Could you check a few things on this model? Use its own coordinates, in mm. A direction names the side the tool comes from. Coordinates: 2 decimals unless noted, no trailing zeros. Order: outer loops, then holes, each group sorted by start corner. A loop starts at its lowest first (then second) coordinate and runs counter-clockwise, first axis right, second up. Notation, with made-up numbers: M 28.5,22 L 86.5,22 A22 cw 86.5,33 Z; hole C -8,47.5 d8. An arc over 180 degrees is marked long. One line per question, with ' | ' between items. Start each with the question number.
from build123d import *

# Parameters (mm, degrees)
F0_R     = 28.575
F1_DEPTH = 40.2336
F2_R     = 3.302
F3_R     = 10.16
F4_DEPTH = 15.7734


with BuildPart() as f1:
    # F0 (on Top) → F1 (new body)
    with BuildSketch(Plane.XY):
        Circle(F0_R)
        with BuildLine():
            ThreePointArc((13.4477648793, -4.826), (-14.2875, 0), (13.4477648793, 4.826))
            Line((13.4477648793, 4.826), (18.5293, 4.826))
            Line((18.5293, 4.826), (18.5293, -4.826))
            Line((18.5293, -4.826), (13.4477648793, -4.826))
        make_face(mode=Mode.SUBTRACT)
    extrude(amount=F1_DEPTH)

    # F2
    f2_edges = [f1.edges().sort_by_distance(p)[0] for p in [
        (-28.575, 0, 40.2336),
    ]]
    fillet(f2_edges, radius=F2_R)

    # F3 (on face) → F4 (join)
    with BuildSketch(Plane(origin=(0, 0, 0), x_dir=(1, 0, 0), z_dir=(0, 0, -1))):
        with BuildLine():
            Line((5.7964106128, -27.9809265216), (57.1919272622, -18.7764181619))
            ThreePointArc((57.1919272622, -18.7764181619), (73.025, 0), (57.1919272622, 18.7764181619))
            Line((57.1919272622, 18.7764181619), (5.7964106128, 27.9809265216))
            ThreePointArc((5.7964106128, 27.9809265216), (22.1603594089, 18.0402077557), (28.575, 0))
            ThreePointArc((28.575, 0), (22.1603594089, -18.0402077557), (5.7964106128, -27.9809265216))
        make_face()
        with Locations((53.975, 0)):
            Circle(F3_R, mode=Mode.SUBTRACT)
    extrude(amount=-F4_DEPTH)


solid = f1.part
(1) For P1, Ø8, axis at x = 33.5, z = 8, coming from the -Y side; P2, Ø4, axis at x = 15, z = 17.5, coming from the -Y side; P3, Ø3, axis at x = 59.5, y = 14, coming from the +Z side, each with a flat end and sliding along its axis, tell me the tip position at first contact or that it passes through.
(2) We'd pull the mould along X, two halves only. Please class faces 1 (the flat face through (18.529, 0, 20)), 2 (the flat face through (16, 4.826, 20)), 3 (the flat face through (22, 0, 0)), 4 (the cylindrical face through (-28.547, 1.256, 22.311)): +X half, -X half, draft (parallel to the pull), parting line (faces both ways), or undercut.
(3) Imagine slicing it at A-A, the plane y = 0. Write out the boundary of the cut face in (x, z) (1 decimal), plus the area to 3 significant figures.
(4) If I drill on line 1 along X through (y, z) = (0, 12) (1 decimal); line 2 along X through (y, z) = (-3, 12); line 3 along Y through (x, z) = (0, 28) (1 decimal), over which ranges is the centre line in solid material (lowest first)? Write a range as from..to.
(5) On a 3-axis mill with a long thin cutter (end or side, diameter ignored), from which of +Z, -Z, +X, -X, +Y, -Y can I reach the whole of each face in a straight line? I mean faces 5 (the flat face through (16, -4.826, 20)), 6 (the flat face through (31.854, -23.314, 7.776)). Say none if no direction works.
(6) Imagine slicing it at D-D, the plane x = 53.5. Write out the boundary of the cut face in (y, z), plus the area to 3 significant figures.
(7) Imagine slicing it at B-B, the plane x = 0. Write out the boundary of the cut face in (y, z) (1 decimal), plus the area to 3 significant figures.
Answers:
1) P1: y = -23.74 | P2: y = -26.51 | P3: z = 15.77
2) face 1: undercut | face 2: undercut | face 3: draft | face 4: parting line
3) outline: M -28.6,0 L -14.3,0 L -14.3,40.2 L -25.3,40.2 A3.3 ccw -28.6,36.9 Z; M 18.5,0 L 43.8,0 L 43.8,15.8 L 28.6,15.8 L 28.6,36.9 A3.3 ccw 25.3,40.2 L 18.5,40.2 Z; M 64.1,0 L 73,0 L 73,15.8 L 64.1,15.8 Z | area: 1,350 mm²
4) line 1: -28.6..-14.3, 18.5..43.8, 64.1..73 | line 2: -28.42..-13.97, 18.53..44.27, 63.68..72.79 | line 3: -28.6..-14.3, 14.3..28.6
5) face 5: +Z, -Z | face 6: +Z, -Z, +X, -Y
6) outline: M -19.44,0 L -10.15,0 L -10.15,15.77 L -19.44,15.77 Z; M 10.15,0 L 19.44,0 L 19.44,15.77 L 10.15,15.77 Z | area: 293 mm²
7) outline: M -28.6,0 L -14.3,0 L -14.3,40.2 L -25.3,40.2 A3.3 ccw -28.6,36.9 Z; M 14.3,0 L 28.6,0 L 28.6,36.9 A3.3 ccw 25.3,40.2 L 14.3,40.2 Z | area: 1,140 mm²
